Read the model definition and answer for the solid it produces. Units are mm, in the model's axes. A direction names the side the tool comes from. Give positions to 0.01 mm unless a question says otherwise; leave off trailing zeros. Write each loop counter-clockwise with the first axis right and the second up, starting at its lowest first coordinate (ties: lowest second). Pieces come first, ordered by that corner, then holes.
```python
from build123d import *

# Parameters (mm, degrees)
SKETCH1_W            = 50.8
SKETCH1_H            = 60.96
BOSS_EXTRUDE2_DEPTH  = 3.175
CUT_EXTRUDE3_DEPTH   = 40.802902218
LPATTERN3_COUNT      = 2
LPATTERN3_PITCH      = 25.4
SKETCH6_R            = 1.5875
CUT_EXTRUDE4_DEPTH   = 40.802902218
MIRROR4_COPY_1_DEPTH = 40.802902218
CUT_EXTRUDE5_DEPTH   = 40.802902218
CUT_EXTRUDE6_DEPTH   = 40.802902218


with BuildPart() as part:
    # Sketch1 → Boss-Extrude2 (new body)
    with BuildSketch(Plane(origin=(0, 0, 0), x_dir=(1, 0, 0), z_dir=(0, 1, 0))):
        Rectangle(SKETCH1_W, SKETCH1_H)
    extrude(amount=BOSS_EXTRUDE2_DEPTH)

    # Sketch5 → Cut-Extrude3 (cut, through all)
    with BuildSketch(Plane(origin=(0, 3.175, 0), x_dir=(1, 0, 0), z_dir=(0, 1, 0))):
        Polygon((-20.32, 6.0325), (-18.415, 6.0325), (-18.415, 7.62), (-15.875, 7.62), (-15.875, 6.0325), (-10.16, 6.0325), (-10.16, 2.8575), (-15.875, 2.8575), (-15.875, 1.27), (-18.415, 1.27), (-18.415, 2.8575), (-20.32, 2.8575), (-20.32, 1.27), (-25.4, 1.27), (-25.4, 7.62), (-20.32, 7.62), align=None)
    cut_extrude3 = extrude(amount=-CUT_EXTRUDE3_DEPTH, mode=Mode.SUBTRACT)

    # LPattern3: Cut-Extrude3 ×2
    with Locations(*[(0, 0, i * LPATTERN3_PITCH) for i in range(1, LPATTERN3_COUNT)]):
        add(cut_extrude3, mode=Mode.SUBTRACT)

    # Sketch6 → Cut-Extrude4 (cut, through all)
    with BuildSketch(Plane(origin=(0, 3.175, 0), x_dir=(1, 0, 0), z_dir=(0, 1, 0))):
        with Locations(Location((-21.9075, -8.255, 0), (0, 0, 270))):
            Circle(SKETCH6_R)
    cut_extrude4 = extrude(amount=-CUT_EXTRUDE4_DEPTH, mode=Mode.SUBTRACT)

    # Mirror4: Cut-Extrude3, Cut-Extrude4 across plane
    add(cut_extrude3.mirror(Plane(origin=(0, 0, 0), x_dir=(0, 0, 1), z_dir=(1, 0, 0))), mode=Mode.SUBTRACT)
    add(cut_extrude4.mirror(Plane(origin=(0, 0, 0), x_dir=(0, 0, 1), z_dir=(1, 0, 0))), mode=Mode.SUBTRACT)

    # Mirror4 copy 1 sketch → Mirror4 copy 1 (cut, through all)
    with BuildSketch(Plane(origin=(0, 3.175, 25.4), x_dir=(-1, 0, 0), z_dir=(0, 1, 0))):
        Polygon((-20.32, -6.0325), (-18.415, -6.0325), (-18.415, -7.62), (-15.875, -7.62), (-15.875, -6.0325), (-10.16, -6.0325), (-10.16, -2.8575), (-15.875, -2.8575), (-15.875, -1.27), (-18.415, -1.27), (-18.415, -2.8575), (-20.32, -2.8575), (-20.32, -1.27), (-25.4, -1.27), (-25.4, -7.62), (-20.32, -7.62), align=None)
    extrude(amount=-MIRROR4_COPY_1_DEPTH, mode=Mode.SUBTRACT)

    # Sketch7 → Cut-Extrude5 (cut, through all)
    with BuildSketch(Plane(origin=(0, 3.175, 0), x_dir=(1, 0, 0), z_dir=(0, 1, 0))):
        Polygon((-3.175, 30.48), (-3.175, 25.4), (-1.5875, 25.4), (-1.5875, 23.495), (-3.175, 23.495), (-3.175, 20.955), (-1.5875, 20.955), (-1.5875, 15.24), (1.5875, 15.24), (1.5875, 20.955), (3.175, 20.955), (3.175, 23.495), (1.5875, 23.495), (1.5875, 25.4), (3.175, 25.4), (3.175, 30.48), align=None)
    extrude(amount=-CUT_EXTRUDE5_DEPTH, mode=Mode.SUBTRACT)

    # Sketch10 → Cut-Extrude6 (cut, through all)
    with BuildSketch(Plane(origin=(0, 3.175, 0), x_dir=(1, 0, 0), z_dir=(0, 1, 0))):
        with BuildLine():
            Line((-25.4, 13.97), (-25.4, 30.48))
            Line((-25.4, 30.48), (-8.89, 30.48))
            ThreePointArc((-8.89, 30.48), (-20.564332957, 25.644332957), (-25.4, 13.97))
        make_face()
        with BuildLine():
            Line((25.4, 13.97), (25.4, 30.48))
            Line((25.4, 30.48), (8.89, 30.48))
            ThreePointArc((8.89, 30.48), (20.564332957, 25.644332957), (25.4, 13.97))
        make_face()
    extrude(amount=-CUT_EXTRUDE6_DEPTH, mode=Mode.SUBTRACT)


solid = part.part
```
Item 1: Determine the mould class of faces 1 (the flat face through (-18.415, 2, -7)), 2 (the flat face through (20.32, 2, -2)), 3 (the flat face through (0, 0, 0)) for opening direction X: pulls with the +X half, pulls with the -X half, needs draft (parallel to the pull), parting line crosses it, or undercut.
Result set:
face 1: undercut
face 2: pulls with the +X half
face 3: needs draft
Item 2: Which of the six approach directions +Z, -Z, +X, -X, +Y, -Y give full straight-line access (tool end or side, diameter ignored) to faces 4 (the flat face through (13, 2, 19.368)), 5 (the flat face through (-20.32, 2, 23)), 6 (the flat face through (2, 2, -20.955)), 7 (the flat face through (1.588, 2, -24))?
Result set:
face 4: +X, +Y, -Y
face 5: -X, +Y, -Y
face 6: +Y, -Y
face 7: -Z, +Y, -Y
Item 3: Section C-C (y = 1) is taken. Give the number of separate pieces and of enclosed holes in the cut face, and give its area (3 significant figures).
Result set:
separate pieces: 1
enclosed holes: 2
area: 2,600 mm2
Item 4: Each of these flat-tipped pins is pushed along its axis until it touches: pin 1 Ø1.7 at (x, y) = (-2, 2) entering from -Z; pin 2 Ø1 at (x, y) = (19.5, 2) entering from -Z; pin 3 Ø1.6 at (x, y) = (-22.5, 1) entering from -Z. Where does it stop, or does it pass through?
Result set:
pin 1: stops at z = -25.4
pin 2: stops at z = -27.02
pin 3: stops at z = -24.39
Item 5: Section A-A (x = -14.5) is taken. Write down the section's boundary in (y, z) (1 decimal), and give its area (3 significant figures).
Result set:
outline: (0, -29.5) - (3.2, -29.5) - (3.2, -6) - (0, -6) - close; (0, -2.9) - (3.2, -2.9) - (3.2, 19.4) - (0, 19.4) - close; (0, 22.5) - (3.2, 22.5) - (3.2, 30.5) - (0, 30.5) - close
area: 170 mm2
Item 6: Section B-B (z = -16) is taken. Write down the section's boundary in (x, y) (1 decimal).
Result set:
outline: (-25.3, 0) - (-1.6, 0) - (-1.6, 3.2) - (-25.3, 3.2) - close; (1.6, 0) - (25.3, 0) - (25.3, 3.2) - (1.6, 3.2) - close
Item 7: Section D-D (z = -5) is taken. Write down the section's boundary in (x, y) (3 decimals).
Result set:
outline: (-10.16, 0) - (10.16, 0) - (10.16, 3.175) - (-10.16, 3.175) - close
Item 8: Find the intervals of material crossed by line 1 along X through (y, z) = (0.2, -7.5) (3 decimals); line 2 along Z through (x, y) = (2, 2) (3 decimals); line 3 along Z through (x, y) = (10.5, 2.5), in increasing order.
Result set:
line 1: x = -20.32 to -18.415, -15.875 to 15.875, 18.415 to 20.32
line 2: z = -25.4 to -23.495, -20.955 to 30.48
line 3: z = -30.4 to -6.03, -2.86 to 19.37, 22.54 to 30.48
